The listing builds one solid part. Answer for the finished solid, in the listing's coordinates (mm). A direction names the side the tool comes from. Round coordinates to 2 decimals unless told otherwise and drop trailing zeros. Write each loop counter-clockwise with the first axis right and the second up, starting at its lowest first coordinate (ties: lowest second). Pieces come first, ordered by that corner, then holes.
Item 1: A tool of negligible diameter and unlimited length cuts with its end or side. For faces 1 (the face through (9.797, -3, -3)), 2 (the face through (11.797, 0, -3)), from which of +Z, -Z, +X, -X, +Y, -Y can it reach the whole face along a straight path? Write none if from no direction.
Item 2: Find section C-C on x = 1.5. Give the vertices of the cut face in (y, z), then the cut area to 3 significant figures.
Item 3: Find section A-A on y = 1. Give the vertices of the cut face in (x, z).
Item 4: Find section B-B on z = -3.25. Give the vertices of the cut face in (x, y), then the cut area to 3 significant figures.
Item 5: Find the intervals of material crossed by probe 1 along Y at (x, z) = (0, -3.5); probe 2 along X at (y, z) = (-2, -1.5); probe 3 along Y at (x, z) = (-6.25, -6.25), in increasing order.
Item 6: This flat-tipped pin is pushed along its axis until it touches: pin 1 (1.5 mm diameter, centred on x = -1.5, z = -2.5, fed in from -Y). Where does it stop, or does it pass through?
Item 7: For a pull along X with two mould halves and no side action, classify faces 3 (the face through (10.94, 6.1, -3.55)), 4 (the face through (0, 0, -3)), 5 (the face through (3, 2, 0)), 6 (the face through (-11.797, 0, -3)) as +X half, -X half, draft (parallel to the pull), parting line (faces both ways), or undercut.
Item 8: Find section D-D on x = 7.25. Give the vertices of the cut face in (y, z), then the cut area to 3 significant figures.
```python
from build123d import *

# Parameters (mm, degrees)
BOSS_EXTRUDE1_DEPTH = 7
SKETCH5_R           = 2.5
CUT_EXTRUDE2_DEPTH  = 16.400080851
FILLET1_R           = 3
FILLET2_R           = 3
FILLET3_R           = 1.5
FILLET4_R           = 1.5


with BuildPart() as part:
    # Sketch1 → Boss-Extrude1 (new body)
    with BuildSketch(Plane.XY):
        Polygon((9.79671523, 0), (-9.79671523, 0), (-9.79671523, -5), (-11.79671523, -5), (-11.79671523, 7), (11.79671523, 7), (11.79671523, -5), (9.79671523, -5), align=None)
    extrude(amount=-BOSS_EXTRUDE1_DEPTH)

    # Sketch5 → Cut-Extrude2 (cut, through all)
    with BuildSketch(Plane.XY):
        with Locations((0, 3)):
            Circle(SKETCH5_R)
    extrude(amount=-CUT_EXTRUDE2_DEPTH, mode=Mode.SUBTRACT)

    # Fillet1
    fillet1_edges = [part.edges().sort_by_distance(p)[0] for p in [
        (11.79671523, 7, -3.5),
    ]]
    fillet(fillet1_edges, radius=FILLET1_R)

    # Fillet2
    fillet2_edges = [part.edges().sort_by_distance(p)[0] for p in [
        (-11.79671523, 7, -3.5),
    ]]
    fillet(fillet2_edges, radius=FILLET2_R)

    # Fillet3
    fillet3_edges = [part.edges().sort_by_distance(p)[0] for p in [
        (11.79671523, -5, -3.5),
    ]]
    fillet(fillet3_edges, radius=FILLET3_R)

    # Fillet4
    fillet4_edges = [part.edges().sort_by_distance(p)[0] for p in [
        (-11.79671523, -5, -3.5),
    ]]
    fillet(fillet4_edges, radius=FILLET4_R)


solid = part.part
```
Check values:
1. face 1: +Z, -Z, -Y
1. face 2: +Z, -Z, +X, +Y, -Y
2. outline: (0, -7) - (1, -7) - (1, 0) - (0, 0) - close; (5, -7) - (7, -7) - (7, 0) - (5, 0) - close
2. area: 21.0 mm2
3. outline: (-11.8, -7) - (-1.5, -7) - (-1.5, 0) - (-11.8, 0) - close; (1.5, -7) - (11.8, -7) - (11.8, 0) - (1.5, 0) - close
4. outline: (-11.8, -3.5) arc R1.5 ccw to (-10.3, -5) - (-9.8, -5) - (-9.8, 0) - (9.8, 0) - (9.8, -5) - (10.3, -5) arc R1.5 ccw to (11.8, -3.5) - (11.8, 4) arc R3 ccw to (8.8, 7) - (-8.8, 7) arc R3 ccw to (-11.8, 4) - close; hole circle Ø5 at (0, 3)
4. area: 161 mm2
5. probe 1: y = 0 to 0.5, 5.5 to 7
5. probe 2: x = -11.8 to -9.8, 9.8 to 11.8
5. probe 3: y = 0 to 7
6. pin 1: stops at y = 0
7. face 3: +X half
7. face 4: undercut
7. face 5: draft
7. face 6: -X half
8. outline: (0, -7) - (7, -7) - (7, 0) - (0, 0) - close
8. area: 49.0 mm2
